Here's how the part is built. I have some questions about the finished solid (model axes, mm). Face numbers are marked on the shaded views. A direction names the side the tool comes from. Give positions to 0.01 mm unless a question says otherwise; leave off trailing zeros. Loops run counter-clockwise (first coordinate to the right, second up) from the corner with the lowest first, then second, coordinate; pieces in that order, holes last. Notation, with made-up numbers: (79, 60.5) - (122, 60.5) arc R21 cw to (122, 74.5) - close; hole circle Ø11 at (-25.5, 2.5). An arc over 180 degrees is marked (long way). Return JSON: item names as keys, results as strings. Group by question number.
(1) On a 3-axis mill with a long thin cutter (end or side, diameter ignored), from which of +Z, -Z, +X, -X, +Y, -Y can I reach the whole of each face in a straight line? I mean the marked faces 1, 2 and 3. Say none if no direction works.
(2) If we section it at A-A (y = -20): Please give me the cut outline in (x, z), then the cut area to 3 significant figures.
(3) For P1, Ø7, axis at x = -30, y = 32.5, coming from the +Z side; P2, Ø5, axis at x = -10.5, z = 25, coming from the -Y side; P3, Ø12, axis at y = -19.5, z = 7.5, coming from the -X side; P4, Ø5.5, axis at x = 0, z = 40, coming from the -Y side, each with a flat end and sliding along its axis, tell me the tip position at first contact or that it passes through.
(4) If we section it at C-C (z = 4.5): Please give me the cut outline in (x, y), then the cut area to 3 significant figures.
(5) I need wall thicknesses on probe 1 along X at (y, z) = (-0.75, 40); probe 2 along X at (y, z) = (-9, 2); probe 3 along Y at (x, z) = (2, 12.5). Which ranges of each line are inside material? Lowest first, please. Write a range as [from, to].
(6) If we mould it in two halves opening along Y, with no side actions, what happens to the marked faces 4, 5 and 6? For each: released by +Y, released by -Y, zero draft, split by the parting line, or undercut.
(7) If we section it at D-D (x = 0): Please give me the cut outline in (y, z), then the cut area to 3 significant figures.
(8) If we section it at B-B (z = 40): Please give me the cut outline in (x, y), then the cut area to 3 significant figures.
```python
from build123d import *

# Parameters (mm, degrees)
SKETCH_1_W          = 30
SKETCH_1_H          = 75
SKETCH_1_R          = 5.5
EXTRUDE_1_DEPTH     = 10
SKETCH_2_W          = 30
SKETCH_2_H          = 15
EXTRUDE_2_DEPTH     = 40
FILLET_1_R          = 2
SKETCH_3_R          = 4.5
CUT_EXTRUDE_1_DEPTH = 15
SKETCH_5_W          = 20
SKETCH_5_H          = 15
EXTRUDE_3_DEPTH     = 30
SKETCH_6_R          = 4.5
CUT_EXTRUDE_2_DEPTH = 30
FILLET_2_R          = 15
SKETCH_7_W          = 20
SKETCH_7_H          = 15
EXTRUDE_4_DEPTH     = 30
FILLET_3_R          = 15
SKETCH_8_R          = 4.5
CUT_EXTRUDE_3_DEPTH = 30
EXTRUDE_5_DEPTH     = 10
FILLET_4_R          = 5
FILLET_5_R          = 10
SKETCH_10_R         = 3.1
CUT_EXTRUDE_4_DEPTH = 10


with BuildPart() as part:
    # 草图1 → 凸台-拉伸1 (new body)
    with BuildSketch(Plane.XY):
        Rectangle(SKETCH_1_W, SKETCH_1_H)
        with Locations((0, 20)):
            Circle(SKETCH_1_R, mode=Mode.SUBTRACT)
        with Locations((0, -20)):
            Circle(SKETCH_1_R, mode=Mode.SUBTRACT)
    extrude(amount=EXTRUDE_1_DEPTH)

    # 草图2 → 凸台-拉伸2 (add)
    with BuildSketch(Plane.XY.offset(10)):
        Rectangle(SKETCH_2_W, SKETCH_2_H)
    extrude(amount=EXTRUDE_2_DEPTH)

    # 圆角1
    fillet_1_edges = [part.edges().sort_by_distance(p)[0] for p in [
        (0, 7.5, 10),
        (0, -7.5, 10),
    ]]
    fillet(fillet_1_edges, radius=FILLET_1_R)

    # 草图3 → 切除-拉伸1 (cut)
    with BuildSketch(Plane(origin=(0, -7.5, 0), x_dir=(-1, 0, 0), z_dir=(0, -1, 0))):
        with Locations((0, -40)):
            Circle(SKETCH_3_R)
    extrude(amount=-CUT_EXTRUDE_1_DEPTH, mode=Mode.SUBTRACT)

    # 草图5 → 凸台-拉伸3 (add)
    with BuildSketch(Plane(origin=(15, 0, 0), x_dir=(0, 0, -1), z_dir=(1, 0, 0))):
        with Locations((-40, 0)):
            Rectangle(SKETCH_5_W, SKETCH_5_H)
    extrude(amount=EXTRUDE_3_DEPTH)

    # 草图6 → 切除-拉伸2 (cut)
    with BuildSketch(Plane(origin=(0, -7.5, 0), x_dir=(-1, 0, 0), z_dir=(0, -1, 0))):
        with Locations((-30, -40)):
            Circle(SKETCH_6_R)
    extrude(amount=-CUT_EXTRUDE_2_DEPTH, mode=Mode.SUBTRACT)

    # 圆角2
    fillet_2_edges = [part.edges().sort_by_distance(p)[0] for p in [
        (15, 0, 30),
    ]]
    fillet(fillet_2_edges, radius=FILLET_2_R)

    # 草图7 → 凸台-拉伸4 (add)
    with BuildSketch(Plane.ZY.offset(15)):
        with Locations((40, 0)):
            Rectangle(SKETCH_7_W, SKETCH_7_H)
    extrude(amount=EXTRUDE_4_DEPTH)

    # 圆角3
    fillet_3_edges = [part.edges().sort_by_distance(p)[0] for p in [
        (-15, 0, 30),
    ]]
    fillet(fillet_3_edges, radius=FILLET_3_R)

    # 草图8 → 切除-拉伸3 (cut)
    with BuildSketch(Plane(origin=(0, -7.5, 0), x_dir=(-1, 0, 0), z_dir=(0, -1, 0))):
        with Locations((30, -40)):
            Circle(SKETCH_8_R)
    extrude(amount=-CUT_EXTRUDE_3_DEPTH, mode=Mode.SUBTRACT)

    # 草图9 → 凸台-拉伸5 (add)
    with BuildSketch(Plane.XY.offset(10)):
        with BuildLine():
            Line((-30, 42.5), (-5, 42.5))
            Line((-5, 42.5), (0, 37.5))
            Line((0, 37.5), (-15, 22.5))
            Line((-15, 22.5), (-30, 22.5))
            ThreePointArc((-30, 22.5), (-40, 32.5), (-30, 42.5))
        make_face()
    extrude(amount=-EXTRUDE_5_DEPTH)

    # 圆角4
    fillet_4_edges = [part.edges().sort_by_distance(p)[0] for p in [
        (-5, 42.5, 5),
        (0, 37.5, 5),
    ]]
    fillet(fillet_4_edges, radius=FILLET_4_R)

    # 圆角5
    fillet_5_edges = [part.edges().sort_by_distance(p)[0] for p in [
        (-15, 22.5, 5),
    ]]
    fillet(fillet_5_edges, radius=FILLET_5_R)

    # 草图10 → 切除-拉伸4 (cut)
    with BuildSketch(Plane.XY.offset(10)):
        with Locations((-30, 32.5)):
            Circle(SKETCH_10_R)
    extrude(amount=-CUT_EXTRUDE_4_DEPTH, mode=Mode.SUBTRACT)


solid = part.part
```
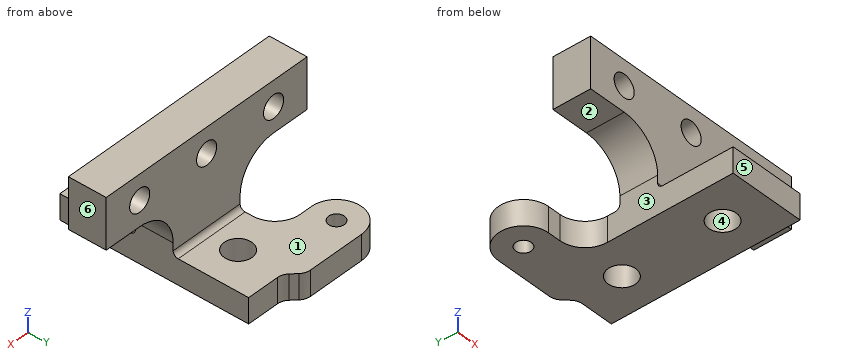
Values:
{
 "1": {"face 1": "+Z, +X, -X, +Y", "face 2": "-Z, -X, +Y, -Y", "face 3": "-Z, -X, -Y"},
 "2": {"outline": "(-15, 0) - (-5.5, 0) - (-5.5, 10) - (-15, 10) - close; (5.5, 0) - (15, 0) - (15, 10) - (5.5, 10) - close", "area": "190 mm2"},
 "3": {"P1": "z = 10", "P2": "y = -7.5", "P3": "x = -15", "P4": "through"},
 "4": {"outline": "(-30, 22.5) - (-25, 22.5) arc R10 cw to (-15, 12.5) - (-15, -37.5) - (15, -37.5) - (15, 37.5) - (2.07, 37.5) arc R5 cw to (-1.46, 38.96) - (-3.54, 41.04) arc R5 ccw to (-7.07, 42.5) - (-30, 42.5) arc R10 ccw to start; hole circle Ø6.2 at (-30, 32.5); hole circle Ø11 at (0, -20); hole circle Ø11 at (0, 20)", "area": "2,570 mm2"},
 "5": {"probe 1": "[-45, -34.5], [-25.5, -4.5], [4.5, 25.5], [34.5, 45]", "probe 2": "[-15, 15]", "probe 3": "[-7.5, 7.5]"},
 "6": {"face 4": "undercut", "face 5": "released by -Y", "face 6": "zero draft"},
 "7": {"outline": "(-37.5, 0) - (-25.5, 0) - (-25.5, 10) - (-37.5, 10) - close; (-14.5, 0) - (14.5, 0) - (14.5, 10) - (9.5, 10) arc R2 cw to (7.5, 12) - (7.5, 35.5) - (-7.5, 35.5) - (-7.5, 12) arc R2 cw to (-9.5, 10) - (-14.5, 10) - close; (-7.5, 44.5) - (7.5, 44.5) - (7.5, 50) - (-7.5, 50) - close; (25.5, 0) - (37.95, 0) - (37.95, 10) - (25.5, 10) - close", "area": "1,000 mm2"},
 "8": {"outline": "(-45, -7.5) - (-34.5, -7.5) - (-34.5, 7.5) - (-45, 7.5) - close; (-25.5, -7.5) - (-4.5, -7.5) - (-4.5, 7.5) - (-25.5, 7.5) - close; (4.5, -7.5) - (25.5, -7.5) - (25.5, 7.5) - (4.5, 7.5) - close; (34.5, -7.5) - (45, -7.5) - (45, 7.5) - (34.5, 7.5) - close", "area": "945 mm2"}
}
